Geometry check sheet. Reference: the model listing, model coordinates, mm. Face numbers are marked on the shaded views. Round coordinates to 2 decimals unless told otherwise and drop trailing zeros. Order: outer loops, then holes, each group sorted by start corner. A loop starts at its lowest first (then second) coordinate and runs counter-clockwise, first axis right, second up. Notation, with made-up numbers: (-29.5, 9.5) - (4.5, 9.5) arc R23 ccw to (4.5, 23.5) - close; hole circle Ø4 at (-11, -11.75). An arc over 180 degrees is marked (long way). One line per question, with ' | ' between items. Start each with the question number.
Q1. Mould release check, pull along X, two halves, no side actions. Record for the marked faces 1, 2 and 3: +X half, -X half, draft (parallel to the pull), parting line (faces both ways), or undercut.
Q2. Sectioned sample at B-B, the plane z = 3.75. Enter the section's corners in (x, y), then the cut area to 3 significant figures.
Q3. Material ranges on line 1 along Z through (x, y) = (-1, 1.75); line 2 along Z through (x, y) = (0, 1); line 3 along Y through (x, z) = (0, -2.6), recorded low to high.
Q4. Gauge pin test, flat ends, axial feed: P1, Ø2, axis at x = -0.5, y = 0.5, coming from the +Z side; P2, Ø3, axis at y = 3.5, z = -2.5, coming from the +X side; P3, Ø5, axis at x = 3.5, z = 1, coming from the +Y side. Record the tip position at first contact, or that the pin passes through.
Q5. Sectioned sample at C-C, the plane z = -2. Enter the section's corners in (x, y).
Q6. Sectioned sample at A-A, the plane z = -3. Enter the section's corners in (x, y), then the cut area to 3 significant figures.
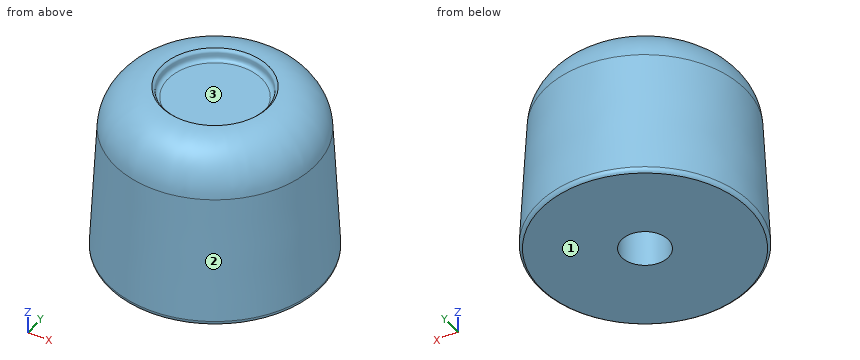
```python
from build123d import *

# Parameters (mm, degrees)
F3_R     = 1.25
F4_DEPTH = 5


with BuildPart() as f2:
    # F1 (on Right) → F2 (revolve)
    with BuildSketch(Plane.YZ):
        with BuildLine():
            Line((-5.3717833243, 2.3256304618), (-5.7258238085, -4.4241435826))
            add(Edge.make_bspline(
                [(-5.7258238085, -4.4241435826), (-5.7264351493, -4.4368966068), (-5.7277565417, -4.464461837), (-5.7161348447, -4.5164232593), (-5.6911095307, -4.5793291163), (-5.6496734627, -4.628407601), (-5.6046093237, -4.659526133), (-5.580468569, -4.6761962585)],
                knots=[0, 0, 0, 0, 0.1612359922, 0.3485061387, 0.5588807728, 0.7636934523, 1, 1, 1, 1], degree=3))
            Line((-5.580468569, -4.6761962585), (0, -4.6761962585))
            Line((0, -4.6761962585), (0, 4.0844450705))
            Line((0, 4.0844450705), (-2.5177469943, 4.0844450705))
            add(Edge.make_bspline(
                [(-2.8773788363, 4.6709873714), (-2.826659029, 4.6275849969), (-2.7331127599, 4.547534807), (-2.7357495643, 4.4104777312), (-2.7417141422, 4.2214380375), (-2.643748447, 4.1210795553), (-2.5745941834, 4.1023556975), (-2.5361450378, 4.0902416719), (-2.5177469943, 4.0844450705)],
                knots=[0, 0, 0, 0, 0.2051585718, 0.3783890356, 0.5853177161, 0.7573058689, 0.8838700543, 1, 1, 1, 1], degree=3))
            ThreePointArc((-2.8773788363, 4.6709873714), (-4.5955361552, 3.999193216), (-5.3717833243, 2.3256304618))
        make_face()
    revolve(axis=Axis((0, 0, -0.295875594), (0, 0, -1)))

    # F3 (on face) → F4 (cut)
    with BuildSketch(Plane(origin=(0, 0, -4.6761962585), x_dir=(1, 0, 0), z_dir=(0, 0, -1))):
        Circle(F3_R)
    extrude(amount=-F4_DEPTH, mode=Mode.SUBTRACT)


solid = f2.part
```
Determined:
1) face 1: draft | face 2: parting line | face 3: undercut
2) outline: circle Ø9.65 at (0, 0) | area: 73.2 mm2
3) line 1: z = -4.68 to 4.08 | line 2: z = 0.32 to 4.08 | line 3: y = -5.63 to -1.25, 1.25 to 5.63
4) P1: stops at z = 4.08 | P2: stops at x = 5.26 | P3: stops at y = 5.37
5) outline: circle Ø11.2 at (0, 0); hole circle Ø2.5 at (0, 0)
6) outline: circle Ø11.3 at (0, 0); hole circle Ø2.5 at (0, 0) | area: 95.4 mm2
